CAD build for the part. Positions are in the model's coordinates, mm. Face numbers are marked on the shaded views. A direction names the side the tool comes from. Coordinates: 2 decimals unless noted, no trailing zeros. Loops run counter-clockwise (first coordinate to the right, second up) from the corner with the lowest first, then second, coordinate; pieces in that order, holes last. Notation, with made-up numbers: (1, 76) -> (10, 76) arc R9 cw to (10, 84) -> close; hole circle Ø1 at (78, 44). An arc over 180 degrees is marked (long way). Write each question's results on one line, items separated by ' | '.
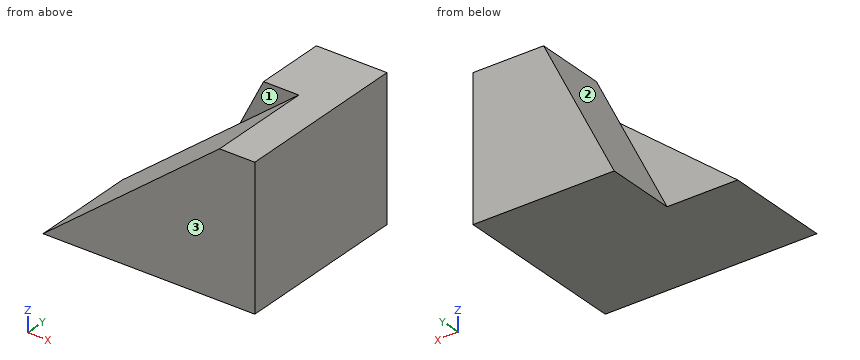
from build123d import *

# Parameters (mm, degrees)
BOSS_EXTRUDE1_DEPTH = 3
BOSS_EXTRUDE2_DEPTH = 4
CUT_EXTRUDE2_DEPTH  = 2


with BuildPart() as part:
    # Sketch1 → Boss-Extrude1 (new body)
    with BuildSketch(Plane(origin=(0, 0, 0), x_dir=(1, 0, 0), z_dir=(0, 1, 0))):
        Polygon((0, 0), (-5, 4), (0, 4), align=None)
    extrude(amount=BOSS_EXTRUDE1_DEPTH)

    # Sketch2 → Boss-Extrude2 (add)
    with BuildSketch(Plane(origin=(0, 0, -4), x_dir=(-1, 0, 0), z_dir=(0, 0, -1))):
        Polygon((1, 5), (3, 5), (3, 3), (0, 3), (0, 0), (-1, 0), (-1, 5), align=None)
    extrude(amount=-BOSS_EXTRUDE2_DEPTH)

    # Sketch4 → Cut-Extrude2 (cut)
    with BuildSketch(Plane(origin=(0, 5, 0), x_dir=(1, 0, 0), z_dir=(0, 1, 0))):
        Polygon((-3, 4), (-1, 0), (-3, 0), align=None)
    extrude(amount=-CUT_EXTRUDE2_DEPTH, mode=Mode.SUBTRACT)


solid = part.part
1) Slice it at B-B (x = -4.6). Write the cut outline in (y, z).
Outcome:
outline: (0, -4) -> (3, -4) -> (3, -3.68) -> (0, -3.68) -> close
2) Drill centre lines: L1, parallel to Y at x = -3.8, z = -3.1; L2, parallel to X at y = 4.3, z = -1.9; L3, parallel to Z at x = -2.5, y = 1.25. Where is each one in solid material? Low to high. Write a range as from..to.
Outcome:
L1: y = 0..3 | L2: x = -1.95..1 | L3: z = -4..-2
3) Slice it at A-A (z = -3.6). Write the cut outline in (x, y).
Outcome:
outline: (-4.5, 0) -> (1, 0) -> (1, 5) -> (-2.8, 5) -> (-2.8, 3) -> (-4.5, 3) -> close
4) Pin check, flat tip, straight feed: pin 1 (1.3 mm diameter, centred on x = -3.5, z = -2.5, fed in from +Y). Stop position of the tip, or through.
Outcome:
pin 1: stops at y = 3
5) Slice it at C-C (y = 4.1). Write the cut outline in (x, z), then the cut area to 3 significant figures.
Outcome:
outline: (-3, -4) -> (1, -4) -> (1, 0) -> (-1, 0) -> close | area: 12.0 mm^2
6) Which spindle directions (+Z, -Z, +X, -X, +Y, -Y) get a long thin tool onto all of the face, cutting with end or side? Do the marked faces 1, 2 and 3. Say none if no direction does.
Outcome:
face 1: +Z, -X, -Y | face 2: +Z, -X, +Y | face 3: +Z, -Z, +X, -X, -Y
